Input: part model. Units: mm. Frame: model coordinates. Face numbers are marked on the shaded views. Coordinates: 2 decimals unless noted, no trailing zeros. Write each loop counter-clockwise with the first axis right and the second up, starting at its lowest first coordinate (ties: lowest second). Pieces come first, ordered by that corner, then holes. Notation, with made-up numbers: (83.25, -32.5) - (120.25, -32.5) arc R24 cw to (120.25, -22.5) - close; hole circle Ø6 at (44, -25.5). An arc over 180 degrees is marked (long way). One line per question, with ' | ' between items. Start each with the question number.
1) Line query: line 1 (Y direction, x = 0, z = -10.25); line 2 (Y direction, x = 0, z = -8.25); line 3 (X direction, y = 2, z = -17.25). Output: solid intervals per line, ascending.
2) Draft query along X for the marked faces 1, 2 and 3. Return one class per face: released by +X, released by -X, zero draft, split by the parting line, or undercut.
3) First-contact query: P1, Ø3, axis at y = -8, z = -18, coming from the +X side; P2, Ø1, axis at x = 12.5, y = 9.5, coming from the -Z side; P3, Ø6, axis at y = -12, z = -15.5, coming from the -X side; P4, Ø8, axis at x = 0, z = -3.5, coming from the -Y side. Flat tips, straight axial feed; report the tip coordinate or a pass-through.
4) Section query A-A on z = -11.5. Return loops of the section in (x, y).
5) Section query B-B on z = -15. Return loops of the section in (x, y), and give its area (3 significant figures).
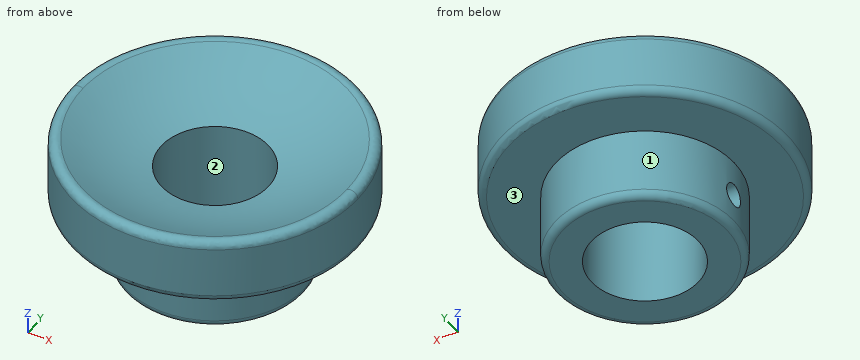
```python
from build123d import *

# Parameters (mm, degrees)
F0_R      = 20
F1_DEPTH  = 10
F4_R      = 12.5
F5_DEPTH  = 10
F6_R      = 1
F8_D      = 15
F10_D     = 3.2
F10_DEPTH = 20.0010001


with BuildPart() as f1:
    # F0 (on Top) → F1 (new body)
    with BuildSketch(Plane.XY):
        Circle(F0_R)
    extrude(amount=-F1_DEPTH)

    # F2 (on Front) → F3 (revolve, cut)
    with BuildSketch(Plane.XZ):
        with BuildLine():
            Line((0, -6), (0, 68))
            ThreePointArc((0, 68), (-37, 31), (0, -6))
        make_face()
    revolve(axis=Axis((0, 0, 31), (0, 0, -1)), mode=Mode.SUBTRACT)

    # F4 (on face) → F5 (join)
    with BuildSketch(Plane(origin=(0, 0, -10), x_dir=(1, 0, 0), z_dir=(0, 0, -1))):
        Circle(F4_R)
    extrude(amount=F5_DEPTH)

    # F6
    f6_edges = [f1.edges().sort_by_distance(p)[0] for p in [
        (0, 20, -0.128765),
        (0, -20, -0.128765),
        (-20, 0, -10),
        (-12.5, 0, -20),
    ]]
    fillet(f6_edges, radius=F6_R)

    # F8 (through all)
    with Locations(Plane(origin=(0, 0, -20), x_dir=(1, 0, 0), z_dir=(0, 0, -1))):
        with Locations((0, 0)):
            Hole(F8_D / 2)

    # F10 (through all, one way)
    with BuildSketch(Plane.YZ):
        with Locations((0, -15)):
            Circle(F10_D / 2)
    extrude(amount=-F10_DEPTH, mode=Mode.SUBTRACT)


solid = f1.part
```
Answer key:
1) line 1: -12.5 to -7.5, 7.5 to 12.5 | line 2: -20 to -7.5, 7.5 to 20 | line 3: -12.34 to -7.23, 7.23 to 12.34
2) face 1: split by the parting line | face 2: undercut | face 3: zero draft
3) P1: x = 10.68 | P2: z = -10 | P3: x = -8.67 | P4: y = -20
4) outline: circle Ø25 at (0, 0); hole circle Ø15 at (0, 0)
5) outline: (-12.4, -1.6) arc R12.5 ccw (long way) to (-12.4, 1.6) - (-7.33, 1.6) arc R7.5 cw (long way) to (-7.33, -1.6) - close | area: 298 mm²
